Geometry check sheet. Reference: the model listing, model coordinates, mm. A direction names the side the tool comes from. Give positions to 0.01 mm unless a question says otherwise; leave off trailing zeros. Order: outer loops, then holes, each group sorted by start corner. A loop starts at its lowest first (then second) coordinate and runs counter-clockwise, first axis right, second up. Notation, with made-up numbers: M -12.75,-30.5 L 8.25,-30.5 A19 cw 8.25,5.5 Z; hole C 37.25,33 d4. An arc over 180 degrees is marked long. Answer as CSV lines item,"result".
from build123d import *

# Parameters (mm, degrees)
F1_DEPTH = 38.1


with BuildPart() as f1:
    # F0 (on Front) → F1 (new body)
    with BuildSketch(Plane.XZ):
        with BuildLine():
            add(Edge.make_bspline(
                [(68.6553490639, 0), (67.8833100518, -1.7748021831), (67.1112710397, -3.5496043662), (66.3392320275, -5.3244065493)],
                knots=[0, 0, 0, 0, 5.8063502503, 5.8063502503, 5.8063502503, 5.8063502503], degree=3))
            add(Edge.make_bspline(
                [(68.6553490639, 0), (68.707247909, 3.4879189514), (68.4529513003, 9.3567744092), (63.2849889631, 13.6707741767), (60.5968596619, 13.4617609131)],
                knots=[0, 0, 0, 0, 0.522788236, 1, 1, 1, 1], degree=3))
            Line((60.5968596619, 13.4617609131), (45.6172116101, 13.6707741767))
            add(Edge.make_bspline(
                [(45.6172116101, 13.6707741767), (43.0083947662, 16.1005357318), (37.5783462559, 21.1578946428), (26.441282578, 27.898149577), (16.7039788369, 29.2117741809), (11.6813281493, 28.8187924523), (9.3536879867, 28.6366734654)],
                knots=[0, 0, 0, 0, 0.26138691, 0.5440564386, 0.7887026968, 1, 1, 1, 1], degree=3))
            Line((9.3536879867, 28.6366734654), (0, 28.6366734654))
            Line((0, 28.6366734654), (-13.6707732454, 28.6366734654))
            Line((-13.6707732454, 28.6366734654), (-13.6707732454, 12.8073561937))
            Line((-13.6707732454, 12.8073561937), (-63.7489780784, 12.8073561937))
            add(Edge.make_bspline(
                [(-63.7489780784, 12.8073561937), (-64.8843970064, 11.6005592617), (-67.4562184604, 8.8670604943), (-69.4633168913, -0.5921410666), (-65.5816661345, -3.8066865274), (-63.7489780784, -5.3244065493)],
                knots=[0, 0, 0, 0, 0.2944087678, 0.6668611617, 1, 1, 1, 1], degree=3))
            Line((-63.7489780784, -5.3244065493), (66.3392320275, -5.3244065493))
        make_face()
    extrude(amount=F1_DEPTH)


solid = f1.part
(1) Section check B-B on x = 49.5. Enter the section's corners in (y, z), then the cut area to 3 significant figures.
The answers:
outline,"M -38.1,-5.32 L 0,-5.32 L 0,13.62 L -38.1,13.62 Z"
area,"722 mm2"
(2) Material ranges on line 1 (Z direction, x = -44, y = -13); line 2 (Z direction, x = -7.5, y = -3); line 3 (X direction, y = -36, z = 2), recorded low to high.
The answers:
line 1,"z = -5.32 to 12.81"
line 2,"z = -5.32 to 28.64"
line 3,"x = -68.35 to 68.66"
(3) Gauge pin test, flat ends, axial feed: P1, Ø6, axis at x = -12.5, y = -11.5, coming from the +Z side; P2, Ø5, axis at x = -25, y = -11, coming from the +Z side; P3, Ø12.5, axis at y = -20, z = 23, coming from the -X side. Record the tip position at first contact, or that the pin passes through.
The answers:
P1,"stops at z = 28.64"
P2,"stops at z = 12.81"
P3,"stops at x = -13.67"
(4) Section check A-A on x = -15.5. Enter the section's corners in (y, z).
The answers:
outline,"M -38.1,-5.32 L 0,-5.32 L 0,12.81 L -38.1,12.81 Z"
(5) Tool access check on faces 1 (the face through (-13.671, -19, 21)), 2 (the face through (1, 0, 8)). Record the directions out of +Z, -Z, +X, -X, +Y, -Y that give a thin tool (end or side, any length) a straight path to the whole face; none if there is none.
The answers:
face 1,"+Z, -X, +Y, -Y"
face 2,"+Z, -Z, +X, -X, +Y"
